Answer from the drawing. Dimensions are ordinates in mm from the lowest x, y and z of the part. A direction names the side the tool comes from. Coordinates: 2 decimals unless noted, no trailing zeros. Write each loop counter-clockwise with the first axis right and the second up, starting at its lowest first coordinate (ties: lowest second). Pieces come first, ordered by that corner, then holes. Notation, with made-up numbers: (-12.75, 17) - (44.25, 17) arc R14 cw to (44.25, 34) - close; hole circle Ø6 at (-2, 49). An arc over 180 degrees is marked (long way). Use a Markdown table: item, result.
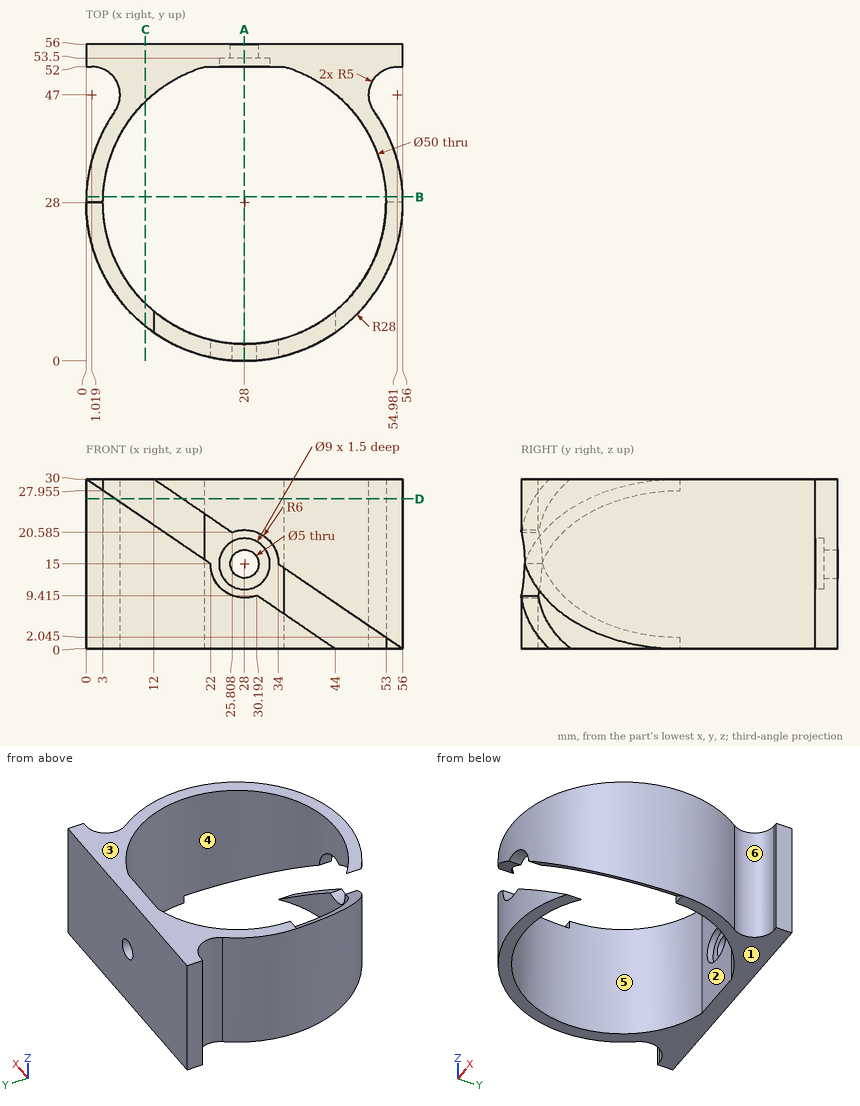
(1) For the marked faces 1 and 2, determine the directions among +Z, -Z, +X, -X, +Y, -Y from which every point of the face is accessible in a straight line to the end or side of a thin tool.
Report:
| item | result |
|---|---|
| face 1 | -Z, +X, -X, +Y, -Y |
| face 2 | +Z, -Z |
(2) Each of these flat-tipped pins is pushed along its axis until it touches: P1, Ø0.6, axis at x = 54, z = 0.5, coming from the -Y side; P2, Ø4.5, axis at x = 27, z = 16, coming from the -Y side; P3, Ø1, axis at x = 2, z = 29, coming from the -Y side (1 decimal). Where does it stop, or does it pass through?
Report:
| item | result |
|---|---|
| P1 | stops at y = 28 |
| P2 | stops at y = 53.5 |
| P3 | stops at y = 17.2 |
(3) Straight lines are drawn through the part: L1, parallel to Z at x = 28, y = 54.9; L2, parallel to X at y = 28, z = 18.5; L3, parallel to X at y = 17.5, z = 4 (1 decimal). For each, find the intervals that lie inside material, in ascending order.
Report:
| item | result |
|---|---|
| L1 | z = 0 to 12.5, 17.5 to 30 |
| L2 | x = 0 to 3, 53 to 56 |
| L3 | x = 2 to 5.3, 50.7 to 54 |
(4) The mould has two halves that part along X. Classify the marked faces 3, 4, 5 and 6: pulls with the +X half, pulls with the -X half, needs draft (parallel to the pull), parting line crosses it, or undercut.
Report:
| item | result |
|---|---|
| face 3 | needs draft |
| face 4 | undercut |
| face 5 | undercut |
| face 6 | pulls with the +X half |
(5) A cutting plane is placed at D-D, the plane z = 26.5. Write down the section's boundary in (x, y) (1 decimal), and give its area (3 significant figures).
Report:
| item | result |
|---|---|
| outline | (0, 52) - (1, 52) arc R5 cw to (5.1, 44.1) arc R28 ccw to (5.1, 11.8) - (5.1, 17.9) arc R25 cw to (21, 52) - (35, 52) arc R25 cw (long way) to (17.1, 5.5) - (17.1, 2.2) arc R28 ccw to (50.9, 44.1) arc R5 cw to (55, 52) - (56, 52) - (56, 56) - (0, 56) - close |
| area | 661 mm² |
(6) A cutting plane is placed at A-A, the plane x = 28. Write down the section's boundary in (y, z), and give its area (3 significant figures).
Report:
| item | result |
|---|---|
| outline | (0, 0) - (3, 0) - (3, 9) - (0, 9) - close; (0, 21) - (3, 21) - (3, 30) - (0, 30) - close; (52, 0) - (56, 0) - (56, 12.5) - (53.5, 12.5) - (53.5, 10.5) - (52, 10.5) - close; (52, 19.5) - (53.5, 19.5) - (53.5, 17.5) - (56, 17.5) - (56, 30) - (52, 30) - close |
| area | 148 mm² |
(7) A cutting plane is placed at C-C, the plane x = 10.5. Write down the section's boundary in (y, z), and give its area (3 significant figures).
Report:
| item | result |
|---|---|
| outline | (6.14, 0) - (10.15, 0) - (10.15, 22.84) - (6.14, 22.84) - close; (45.85, 0) - (56, 0) - (56, 30) - (45.85, 30) - close |
| area | 396 mm² |
(8) A cutting plane is placed at B-B, the plane y = 29. Write down the section's boundary in (x, z).
Report:
| item | result |
|---|---|
| outline | (0.02, 0) - (3.02, 0) - (3.02, 30) - (0.02, 30) - close; (52.98, 0) - (55.98, 0) - (55.98, 30) - (52.98, 30) - close |
